Source: CAD feature listing. Evaluate the final solid. Frame: model axes, mm. Coordinates: 2 decimals unless noted, no trailing zeros. Write each loop counter-clockwise with the first axis right and the second up, starting at its lowest first coordinate (ties: lowest second). Pieces come first, ordered by that corner, then holes. Notation, with made-up numbers: (-25, -14) - (13, -14) arc R11 cw to (13, 4) - close; hole circle Ø1 at (-8.75, 24). An arc over 180 degrees is marked (long way). One line per question, with ' | ' between items. Start each with the question number.
Q1. Cut plane A-A, the plane x = -6.75. Give the number of separate pieces and of enclosed holes in the cut face, plus the area to 3 significant figures.
Q2. Contact query for flat-ended pins moving along their axis: P1, Ø2, axis at y = 6.5, z = 31.5, coming from the +X side; P2, Ø3, axis at x = -6.5, z = 33, coming from the +Y side; P3, Ø3, axis at x = -2, z = 32, coming from the -Y side; P4, Ø2, axis at y = 1, z = 33.5, coming from the +X side. Output: stop coordinate, or through.
Q3. Cut plane C-C, the plane y = -9. Return loops of the section in (x, z), plus the area to 3 significant figures.
Q4. Line query: line 1 (X direction, y = -6.5, z = 31.9); line 2 (Y direction, x = -7.25, z = 31); line 3 (Y direction, x = -6.75, z = 32.85). Output: solid intervals per line, ascending.
Q5. Draft query along Y for faces 1 (the face through (-5, 5, 35)), 2 (the face through (3.573, 5.626, 33.038)). Return one class per face: +Y half, -Y half, draft (parallel to the pull), parting line (faces both ways), or undercut.
```python
from build123d import *

# Parameters (mm, degrees)
PAD016_DEPTH          = 5
POLARPATTERN013_COUNT = 10


with BuildPart() as part:
    # Sketch022 → Pad016 (new body)
    with BuildSketch(Plane.XY):
        with BuildLine():
            ThreePointArc((4.319673, 10.116344), (0, 11), (-4.319673, 10.116344))
            Line((-0.844746, 5.333517), (-4.319673, 10.116344))
            Line((0, 7.933378), (-0.844746, 5.333517))
            Line((0, 7.933378), (0.844746, 5.333517))
            Line((4.319673, 10.116344), (0.844746, 5.333517))
        make_face()
    pad016 = extrude(amount=PAD016_DEPTH)

    # PolarPattern013: Pad016 ×10 about axis
    polarpattern013_axis = Axis((0, 0, 0), (0, 0, 1))
    for i in range(1, POLARPATTERN013_COUNT):
        add(pad016.rotate(polarpattern013_axis, i * 360 / POLARPATTERN013_COUNT))

    # Cone003 → Cone003 (revolve, cut)
    with BuildSketch(Plane(origin=(0, 0, 2), x_dir=(-1, 0, 0), z_dir=(0, -1, 0))):
        Polygon((0, 0), (5, 0), (8, 2), (0, 2), align=None)
    revolve(axis=Axis((0, 0, 2), (0, 0, -1)), mode=Mode.SUBTRACT)


with BuildPart() as part_1:
    # Body028 placement: moved
    add(part.part.moved(Location((0, 0, 30))))


solid = part_1.part
```
Reply:
1) separate pieces: 4 | enclosed holes: 0 | area: 73.9 mm^2
2) P1: stops at x = 9.53 | P2: stops at y = 9.8 | P3: stops at y = -10.99 | P4: stops at x = 11
3) outline: (-6.32, 30) - (6.32, 30) - (6.32, 35) - (-6.32, 35) - close | area: 63.2 mm^2
4) line 1: x = -8.87 to -2.45, -1.69 to -0.47, 0.47 to 1.69, 2.45 to 8.87 | line 2: y = -8.27 to -2.45, -2.24 to -0.22, 0.22 to 2.24, 2.45 to 8.27 | line 3: y = -8.69 to -2.45, -1.87 to -0.38, 0.38 to 1.87, 2.45 to 8.69
5) face 1: draft | face 2: undercut
